from build123d import *

# Parameters (mm, degrees)
EXTRUDE_START       = 50
SKETCH_1_R          = 20
SKETCH_1_R_2        = 11
EXTRUDE_1_DEPTH     = 15
SKETCH_2_R          = 32.5
SKETCH_2_R_2        = 10.9
EXTRUDE_2_DEPTH     = 8
SKETCH_3_R          = 2
CUT_EXTRUDE_3_DEPTH = 49.347699015


with BuildPart() as part:
    # Эскиз1 → Вытянуть1 (new body)
    with BuildSketch(Plane.XY.offset(EXTRUDE_START)):
        Circle(SKETCH_1_R)
        Circle(SKETCH_1_R_2, mode=Mode.SUBTRACT)
    extrude(amount=EXTRUDE_1_DEPTH)

    # Эскиз2 → Вытянуть2 (add)
    with BuildSketch(Plane.XY.offset(65)):
        Circle(SKETCH_2_R)
        Circle(SKETCH_2_R_2, mode=Mode.SUBTRACT)
    extrude(amount=EXTRUDE_2_DEPTH)

    # Эскиз3 → Вытянуть3 (cut, through all)
    with BuildSketch(Plane(origin=(0, 0, 65), x_dir=(-1, 0, 0), z_dir=(0, 0, -1))):
        with Locations((0, 26.5)):
            Circle(SKETCH_3_R)
        with Locations((22.9496732, 13.25)):
            Circle(SKETCH_3_R)
        with Locations((22.9496732, -13.25)):
            Circle(SKETCH_3_R)
        with Locations((0, -26.5)):
            Circle(SKETCH_3_R)
        with Locations((-22.9496732, -13.25)):
            Circle(SKETCH_3_R)
        with Locations((-22.9496732, 13.25)):
            Circle(SKETCH_3_R)
    extrude(amount=-CUT_EXTRUDE_3_DEPTH, mode=Mode.SUBTRACT)


solid = part.part
Can you work these out from the model? Positions are in its coordinate system, mm. A direction names the side the tool comes from. Give positions to 0.01 mm unless a question says otherwise; leave off trailing zeros. Order: outer loops, then holes, each group sorted by start corner. A loop starts at its lowest first (then second) coordinate and runs counter-clockwise, first axis right, second up. Notation, with made-up numbers: M 77,67 L 88,67 A11 cw 88,87 Z; hole C 2.5,-36.75 d4. An arc over 180 degrees is marked long. Use a Markdown table: item, result. Add a question column.
Item 1: Will these pins go through, and if not, where does the flat tip stop? pin 1 (3.5 mm diameter, centred on x = 22.95, y = -13.25, fed in from +Z); pin 2 (2 mm diameter, centred on y = -5.5, z = 62, fed in from +X); pin 3 (4.5 mm diameter, centred on x = -22.95, y = 13.25, fed in from -Z); pin 4 (10 mm diameter, centred on y = 25.5, z = 68, fed in from +X).
Item 2: We'd pull the mould along Y, two halves only. Please class faces 1 (the flat face through (14, 0, 73)), 2 (the cylindrical face through (-4.336, -19.524, 57.395)), 3 (the cylindrical face through (-2.38, -10.74, 57.4)): +Y half, -Y half, draft (parallel to the pull), parting line (faces both ways), or undercut.
Item 3: If I drill on L1, parallel to Y at x = 23.5, z = 66; L2, parallel to Y at x = 0, z = 69.75; L3, parallel to Y at x = 0, z = 59, over which ranges is the centre line in solid material (lowest first)? Write a range as [from, to].
Item 4: For faces 4 (the cylindrical face through (23.21, -11.267, 68.944)), 5 (the flat face through (14, 15, 65)), which set-ups out of +Z, -Z, +X, -X, +Y, -Y let a thin tool reach every point of the face, with its end or its side?
Item 5: Suppose I cut it at B-B (x = 0). List the corners of the cut face in (y, z) for me, then the cut area to 3 significant figures.
Item 6: Suppose I cut it at D-D (x = -23.5). List the corners of the cut face in (y, z) for me.
Item 7: Suppose I cut it at A-A (y = 0). List the corners of the cut face in (x, z) for me, then the cut area to 3 significant figures.
Item 8: Suppose I cut it at C-C (z = 69). List the corners of the cut face in (x, y) for me.
Answer sheet:
| question | item | result |
|---|---|---|
| 1 | pin 1 | passes through |
| 1 | pin 2 | stops at x = 19.49 |
| 1 | pin 3 | stops at z = 65 |
| 1 | pin 4 | stops at x = 25.22 |
| 2 | face 1 | draft |
| 2 | face 2 | parting line |
| 2 | face 3 | undercut |
| 3 | L1 | y = [-22.45, -15.17], [-11.33, 11.33], [15.17, 22.45] |
| 3 | L2 | y = [-32.5, -28.5], [-24.5, -10.9], [10.9, 24.5], [28.5, 32.5] |
| 3 | L3 | y = [-20, -11], [11, 20] |
| 4 | face 4 | +Z, -Z |
| 4 | face 5 | -Z |
| 5 | outline | M -32.5,65 L -28.5,65 L -28.5,73 L -32.5,73 Z; M -24.5,65 L -20,65 L -20,50 L -11,50 L -11,65 L -10.9,65 L -10.9,73 L -24.5,73 Z; M 10.9,65 L 11,65 L 11,50 L 20,50 L 20,65 L 24.5,65 L 24.5,73 L 10.9,73 Z; M 28.5,65 L 32.5,65 L 32.5,73 L 28.5,73 Z |
| 5 | area | 552 mm² |
| 6 | outline | M -22.45,65 L -15.17,65 L -15.17,73 L -22.45,73 Z; M -11.33,65 L 11.33,65 L 11.33,73 L -11.33,73 Z; M 15.17,65 L 22.45,65 L 22.45,73 L 15.17,73 Z |
| 7 | outline | M -32.5,65 L -20,65 L -20,50 L -11,50 L -11,65 L -10.9,65 L -10.9,73 L -32.5,73 Z; M 10.9,65 L 11,65 L 11,50 L 20,50 L 20,65 L 32.5,65 L 32.5,73 L 10.9,73 Z |
| 7 | area | 616 mm² |
| 8 | outline | C 0,0 d65; hole C -22.95,-13.25 d4; hole C -22.95,13.25 d4; hole C 0,0 d21.8; hole C 0,-26.5 d4; hole C 0,26.5 d4; hole C 22.95,-13.25 d4; hole C 22.95,13.25 d4 |
